Verification items for the finished model (mm, model axes). Face numbers are marked on the shaded views. Coordinates: 2 decimals unless noted, no trailing zeros. Order: outer loops, then holes, each group sorted by start corner. A loop starts at its lowest first (then second) coordinate and runs counter-clockwise, first axis right, second up. Notation, with made-up numbers: M -8.75,-24 L 43.25,-24 A16 ccw 43.25,4 Z; hole C 1,-35 d2. An arc over 180 degrees is marked long. Return JSON: item names as keys, results as strings.
```python
from build123d import *

# Parameters (mm, degrees)
SKETCH_1_R          = 15
SKETCH_1_R_2        = 1.45
SKETCH_1_R_3        = 1.5
EXTRUDE_1_DEPTH     = 8
SKETCH_2_R          = 1.45
SKETCH_2_R_2        = 1.5
EXTRUDE_2_DEPTH     = 6
CHAMFER_1_SIZE      = 1.55
SKETCH_3_R          = 1.5
CUT_EXTRUDE_1_DEPTH = 40.846349976
SKETCH_4_R          = 1.5
CUT_EXTRUDE_2_DEPTH = 40.846349976


with BuildPart() as part:
    # 草图1 → 凸台-拉伸1 (new body)
    with BuildSketch(Plane(origin=(0, 0, 0), x_dir=(1, 0, 0), z_dir=(0, 1, 0))):
        Circle(SKETCH_1_R)
        with Locations((0, 12)):
            Circle(SKETCH_1_R_2, mode=Mode.SUBTRACT)
        with Locations((-10.392304845, -6)):
            Circle(SKETCH_1_R_2, mode=Mode.SUBTRACT)
        with Locations((10.392304845, -6)):
            Circle(SKETCH_1_R_2, mode=Mode.SUBTRACT)
        with Locations((-11.258330249, 6.5)):
            Circle(SKETCH_1_R_3, mode=Mode.SUBTRACT)
        with Locations((0, -13)):
            Circle(SKETCH_1_R_3, mode=Mode.SUBTRACT)
        with Locations((11.258330249, 6.5)):
            Circle(SKETCH_1_R_3, mode=Mode.SUBTRACT)
    extrude(amount=EXTRUDE_1_DEPTH)

    # 草图2 → 凸台-拉伸2 (add)
    with BuildSketch(Plane(origin=(0, 8, 0), x_dir=(1, 0, 0), z_dir=(0, 1, 0))):
        with BuildLine():
            Line((-6.859687774, 18.906207542), (15.363533928, 12.979284466))
            ThreePointArc((15.363533928, 12.979284466), (18.402280708, 10.653197849), (18.906207542, 6.859687774))
            Line((18.906207542, 6.859687774), (12.979284466, -15.363533928))
            ThreePointArc((12.979284466, -15.363533928), (10.653197849, -18.402280708), (6.859687774, -18.906207542))
            Line((6.859687774, -18.906207542), (-15.363533928, -12.979284466))
            ThreePointArc((-15.363533928, -12.979284466), (-18.402280708, -10.653197849), (-18.906207542, -6.859687774))
            Line((-18.906207542, -6.859687774), (-12.979284466, 15.363533928))
            ThreePointArc((-12.979284466, 15.363533928), (-10.653197849, 18.402280708), (-6.859687774, 18.906207542))
        make_face()
        with Locations((0, 12)):
            Circle(SKETCH_2_R, mode=Mode.SUBTRACT)
        with Locations((-11.258330249, 6.5)):
            Circle(SKETCH_2_R_2, mode=Mode.SUBTRACT)
        with Locations((11.258330249, 6.5)):
            Circle(SKETCH_2_R_2, mode=Mode.SUBTRACT)
        with Locations((-10.392304845, -6)):
            Circle(SKETCH_2_R, mode=Mode.SUBTRACT)
        with Locations((0, -13)):
            Circle(SKETCH_2_R_2, mode=Mode.SUBTRACT)
        with Locations((10.392304845, -6)):
            Circle(SKETCH_2_R, mode=Mode.SUBTRACT)
    extrude(amount=-EXTRUDE_2_DEPTH)

    # 倒角1
    chamfer_1_edges = [part.edges().sort_by_distance(p)[0] for p in [
        (8.942304845, 8, 6),
        (-1.45, 8, -12),
        (-11.842304845, 8, 6),
    ]]
    chamfer(chamfer_1_edges, length=CHAMFER_1_SIZE)

    # 草图3 → 切除-拉伸1 (cut, through all)
    with BuildSketch(Plane(origin=(-15.942746004, 0, -4.251923077), x_dir=(-0.257692308, 0, 0.966227031), z_dir=(-0.966227031, 0, -0.257692308))):
        with Locations((0, 5)):
            Circle(SKETCH_3_R)
    extrude(amount=-CUT_EXTRUDE_1_DEPTH, mode=Mode.SUBTRACT)

    # 草图4 → 切除-拉伸2 (cut, through all)
    with BuildSketch(Plane(origin=(4.251923077, 0, -15.942746004), x_dir=(-0.966227031, 0, -0.257692308), z_dir=(0.257692308, 0, -0.966227031))):
        with Locations((0.092307692, 5)):
            Circle(SKETCH_4_R)
    extrude(amount=-CUT_EXTRUDE_2_DEPTH, mode=Mode.SUBTRACT)


solid = part.part
```
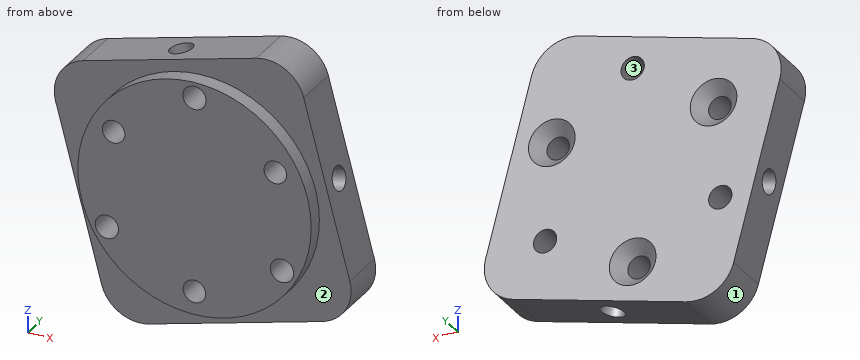
Q1. Material ranges on line 1 along Z through (x, y) = (0, 1.75); line 2 along X through (y, z) = (3.25, 6); line 3 along X through (y, z) = (3.75, 6), recorded low to high.
Values:
{"line 1": "-15 to -13.45, -10.55 to 11.5, 14.5 to 15", "line 2": "-18.68 to -11.84, -8.94 to 8.94, 11.84 to 15.48", "line 3": "-18.68 to -11.84, -8.94 to -2.55, -0.84 to 8.94, 11.84 to 15.48"}
Q2. Go/stop test with flat-tipped pins: pin 1 (1.8 mm diameter, centred on x = -11.26, z = -6.5, fed in from +Y); pin 2 (1.5 mm diameter, centred on x = -10.5, z = 4.5, fed in from +Y); pin 3 (4 mm diameter, centred on x = -10.39, z = 6, fed in from +Y); pin 4 (3.5 mm diameter, centred on x = 0, z = -12, fed in from +Y). Record where each tip stops, or that it passes through.
Values:
{"pin 1": "through", "pin 2": "y = 7.25", "pin 3": "y = 7", "pin 4": "y = 6.75"}
Q3. Draft check along X on the marked faces 1, 2 and 3. Enter one of: pulls with the +X half, pulls with the -X half, needs draft (parallel to the pull), parting line crosses it, or undercut.
Values:
{"face 1": "parting line crosses it", "face 2": "needs draft", "face 3": "undercut"}
Q4. Cross-section at A-A, the plane y = 5.5. State how many separate pieces and enclosed holes the cut face has, and give its area (3 significant figures).
Values:
{"separate pieces": "4", "enclosed holes": "6", "area": "848 mm^2"}
Q5. Cross-section at B-B, the plane y = 7.5. Record the boundary of the cut face in (x, z), and give its area (3 significant figures).
Values:
{"outline": "M -18.91,6.86 L -12.98,-15.36 A5 ccw -6.86,-18.91 L 15.36,-12.98 A5 ccw 18.91,-6.86 L 12.98,15.36 A5 ccw 6.86,18.91 L -15.36,12.98 A5 ccw Z; hole C -10.39,6 d5; hole C -11.26,-6.5 d3; hole C 0,-12 d5; hole C 0,13 d3; hole C 10.39,6 d5; hole C 11.26,-6.5 d3", "area": "987 mm^2"}
